Model file for the job. Use its own axes, mm. A direction names the side the tool comes from. Coordinates: 2 decimals unless noted, no trailing zeros. Write each loop counter-clockwise with the first axis right and the second up, starting at its lowest first coordinate (ties: lowest second). Pieces come first, ordered by that corner, then holes. Notation, with made-up numbers: (55.25, -14) -> (89.25, -14) arc R24 cw to (89.25, 3) -> close; hole circle Ø6 at (3.5, 16.5). An arc over 180 degrees is marked (long way). Answer as a JSON object with one key per item and string values. Group by question number.
from build123d import *

# Parameters (mm, degrees)
SKETCH_2_OUTSIDE_W       = 57.368
SKETCH_2_OUTSIDE_H       = 57.368
CUT_EXTRUDE_1_DEPTH      = 41.509258201
SKETCH_3_OUTSIDE_W       = 188.496
SKETCH_3_OUTSIDE_H       = 193.138
SKETCH_3_OUTSIDE_R       = 15
CUT_EXTRUDE_2_DEPTH      = 41.174618853
CUT_EXTRUDE_2_DRAFT      = -60
SKETCH_4_OUTSIDE_W       = 177.358
SKETCH_4_OUTSIDE_H       = 182
SKETCH_4_OUTSIDE_R       = 14
CUT_EXTRUDE_3_DEPTH      = 37.959437225
CUT_EXTRUDE_3_DRAFT      = -60
SKETCH_5_R               = 0.75
CUT_EXTRUDE_4_DEPTH      = 57.824290581
PATTERN_CIRCULAR_1_COUNT = 3


with BuildPart() as part:
    # Эскиз1 → Повернуть1 (revolve)
    with BuildSketch(Plane.XY):
        with BuildLine():
            Line((0, 7.75), (-19.3, 7.75))
            Line((-19.3, 7.75), (-19.3, 3))
            Line((-19.3, 3), (-52, 3))
            Line((-52, 3), (-52, 6.75))
            Line((-52, 6.75), (-51.75, 7))
            Line((-51.75, 7), (-49, 7))
            Line((-49, 7), (-49, 12.4))
            Line((-49, 12.4), (-46, 12.4))
            Line((-46, 12.4), (-44.9, 13.5))
            Line((-44.9, 13.5), (-33.3, 13.5))
            Line((-33.3, 13.5), (-32.419669914, 12.619669914))
            ThreePointArc((-32.419669914, 12.619669914), (-32.176352402, 12.457090351), (-31.889339828, 12.4))
            Line((-31.889339828, 12.4), (-29.75, 12.4))
            ThreePointArc((-29.75, 12.4), (-29.219669914, 12.619669914), (-29, 13.15))
            Line((-29, 13.15), (-29, 20))
            Line((-29, 20), (-19, 20))
            Line((-19, 20), (-19, 15))
            Line((-19, 15), (-17, 15))
            Line((-17, 15), (-17, 12))
            Line((-17, 12), (-14, 12))
            Line((-14, 12), (-14, 11.6))
            ThreePointArc((-14, 11.6), (-13.780330086, 11.069669914), (-13.25, 10.85))
            Line((-13.25, 10.85), (-11.110660172, 10.85))
            ThreePointArc((-11.110660172, 10.85), (-10.823647598, 10.907090351), (-10.580330086, 11.069669914))
            Line((-10.580330086, 11.069669914), (-9.65, 12))
            Line((-9.65, 12), (-1.6, 12))
            Line((-1.6, 12), (0, 10.4))
            Line((0, 10.4), (0, 7.75))
        make_face()
    revolve(axis=Axis((0, 0, 0), (-1, 0, 0)))

    # Эскиз2 outside → Вырез-Вытянуть1 (cut, through all)
    with BuildSketch(Plane.ZY.offset(29)):
        Rectangle(SKETCH_2_OUTSIDE_W, SKETCH_2_OUTSIDE_H)
        Polygon((0, 17.320508076), (-15, 8.660254038), (-15, -8.660254038), (0, -17.320508076), (15, -8.660254038), (15, 8.660254038), align=None, mode=Mode.SUBTRACT)
    extrude(amount=-CUT_EXTRUDE_1_DEPTH, mode=Mode.SUBTRACT)


with BuildPart() as cut_extrude_2_tool:
    # Эскиз3 outside → Вырез-Вытянуть2 (with draft: the straight prism first)
    with BuildSketch(Plane(origin=(-19, 0, 0), x_dir=(0, 0, -1), z_dir=(1, 0, 0))):
        Rectangle(SKETCH_3_OUTSIDE_W, SKETCH_3_OUTSIDE_H)
        with Locations(Location((0, 0, 0), (0, 0, 90))):
            Circle(SKETCH_3_OUTSIDE_R, mode=Mode.SUBTRACT)
    extrude(amount=-CUT_EXTRUDE_2_DEPTH)
    # Вырез-Вытянуть2: the draft: its side faces are tilted about the plane it starts from
    cut_extrude_2_sides = [cut_extrude_2_tool.faces().sort_by_distance(p)[0] for p in [
        (-39.587309427, -96.569, 0),
        (-39.587309427, 0, -94.248),
        (-39.587309427, 96.569, 0),
        (-39.587309427, 0, 94.248),
        (-39.587309427, -15, 0),
    ]]
    draft(cut_extrude_2_sides, Plane(origin=(-19, 0, 0), x_dir=(0, 0, -1), z_dir=(1, 0, 0)), CUT_EXTRUDE_2_DRAFT)


with BuildPart() as part_1:
    add(part.part)

    # Вырез-Вытянуть2: cut by cut_extrude_2_tool
    add(cut_extrude_2_tool.part, mode=Mode.SUBTRACT)


with BuildPart() as cut_extrude_3_tool:
    # Эскиз4 outside → Вырез-Вытянуть3 (with draft: the straight prism first)
    with BuildSketch(Plane.ZY.offset(29)):
        Rectangle(SKETCH_4_OUTSIDE_W, SKETCH_4_OUTSIDE_H)
        Circle(SKETCH_4_OUTSIDE_R, mode=Mode.SUBTRACT)
    extrude(amount=-CUT_EXTRUDE_3_DEPTH)
    # Вырез-Вытянуть3: the draft: its side faces are tilted about the plane it starts from
    cut_extrude_3_sides = [cut_extrude_3_tool.faces().sort_by_distance(p)[0] for p in [
        (-10.020281387, -91, 0),
        (-10.020281387, 0, 88.679),
        (-10.020281387, 91, 0),
        (-10.020281387, 0, -88.679),
        (-10.020281387, 0, -14),
    ]]
    draft(cut_extrude_3_sides, Plane.ZY.offset(29), CUT_EXTRUDE_3_DRAFT)


with BuildPart() as part_2:
    add(part_1.part)

    # Вырез-Вытянуть3: cut by cut_extrude_3_tool
    add(cut_extrude_3_tool.part, mode=Mode.SUBTRACT)

    # Эскиз5 → Вырез-Вытянуть4 (cut, symmetric)
    with BuildSketch(Plane.XY):
        with Locations(Location((-24, 13.5, 0), (0, 0, 270))):
            Circle(SKETCH_5_R)
    cut_extrude_4 = extrude(amount=CUT_EXTRUDE_4_DEPTH, both=True, mode=Mode.SUBTRACT)

    # Круговой массив1: Вырез-Вытянуть4 ×3 about axis
    pattern_circular_1_axis = Axis((0, 0, 0), (1, 0, 0))
    for i in range(1, PATTERN_CIRCULAR_1_COUNT):
        add(cut_extrude_4.rotate(pattern_circular_1_axis, i * 360 / PATTERN_CIRCULAR_1_COUNT), mode=Mode.SUBTRACT)


solid = part_2.part
(1) Cut at A-A on x = -24. List the corners of the cut face in (y, z).
(2) Pin check, flat tips, straight feed: pin 1 (12 mm diameter, centred on x = -9.5, z = -10.5, fed in from -Y); pin 2 (1.5 mm diameter, centred on x = -6, y = 0.5, fed in from +Z); pin 3 (3 mm diameter, centred on y = -12.5, z = -2.5, fed in from -X); pin 4 (3.5 mm diameter, centred on y = 0, z = 0, fed in from +X). Stop position of each tip, or through.
(3) Cut at B-B on x = -3.5. List the corners of the cut face in (y, z).
(4) 3-axis set-ups, long thin cutter, end or side, ignore diameter. For faces 4 (the face through (-23, 0, 15)), 5 (the face through (-5.57, -11.99, -0.53)), 6 (the face through (-30.8, 5.72, 11)), 7 (the face through (-49, -5.3, 5.3)): which of +Z, -Z, +X, -X, +Y, -Y reach the whole face in a straight line?
(5) Wall check: probe 1 along Y at (x, z) = (-24, 0); probe 2 along Y at (x, z) = (-42, 0). Give the ranges that are in metal, low to high.
(6) Cut at C-C on z = -1. Give the number of separate pieces and of enclosed holes in the cut face, plus the area to 3 significant figures.
(7) Pull direction Y, two halves, no side cores. Call faces 1 (the face through (-36, -3, 0)), 2 (the face through (-25, 0, -15)), 3 (the face through (-15.48, -11.99, -0.53)): released by +Y, released by -Y, zero draft, split by the parting line, or undercut.
Results found:
{
 "1": {"outline": "(-17.32, 0) -> (-13.23, -7.08) -> (0.48, -15) -> (8.66, -15) -> (12.75, -7.92) -> (12.75, 7.92) -> (8.66, 15) -> (0.48, 15) -> (-13.23, 7.08) -> close; (-11.73, -9.68) -> (-8.66, -15) -> (-2.52, -15) -> close; (-11.73, 9.68) -> (-2.52, 15) -> (-8.66, 15) -> close; (14.25, -5.32) -> (17.32, 0) -> (14.25, 5.32) -> close; hole circle Ø6 at (0, 0)"},
 "2": {"pin 1": "stops at y = -11.12", "pin 2": "stops at z = 12", "pin 3": "stops at x = -49", "pin 4": "passes through"},
 "3": {"outline": "circle Ø24 at (0, 0); hole circle Ø15.5 at (0, 0)"},
 "4": {"face 4": "+Z, +X, -X, +Y, -Y", "face 5": "+X", "face 6": "none", "face 7": "-X"},
 "5": {"probe 1": "y = -17.32 to -3, 3 to 12.75, 14.25 to 17.32", "probe 2": "y = -13.5 to -3, 3 to 13.5"},
 "6": {"separate pieces": "2", "enclosed holes": "1", "area": "865 mm²"},
 "7": {"face 1": "undercut", "face 2": "zero draft", "face 3": "split by the parting line"}
}
